Design review of the part built by this model. Coordinates are the model's own, in mm. A direction names the side the tool comes from. Coordinates: 2 decimals unless noted, no trailing zeros. Write each loop counter-clockwise with the first axis right and the second up, starting at its lowest first coordinate (ties: lowest second). Pieces come first, ordered by that corner, then holes. Notation, with made-up numbers: (85, 10) - (116, 10) arc R29 ccw to (116, 40) - close; hole circle Ø9 at (-28.75, 23). An arc over 180 degrees is marked (long way). One line per item, written item: value.
from build123d import *

# Parameters (mm, degrees)
SWEEP2_PROFILE_R     = 31.5
BOSS_EXTRUDE2_DEPTH  = 21
CUT_EXTRUDE4_REACH   = 47.019
SWEEP4_PROFILE_R     = 17.5
CUT_EXTRUDE5_START   = 2.5
CUT_EXTRUDE5_DEPTH   = 18.5
BOSS_EXTRUDE5_START  = 21
SKETCH47_R           = 5
BOSS_EXTRUDE5_DEPTH  = 7
BOSS_EXTRUDE6_START  = -21
SKETCH47_3_R         = 5
BOSS_EXTRUDE6_DEPTH  = 7
CUT_SWEEP1_PROFILE_R = 26
CUT_SWEEP2_PROFILE_R = 12


with BuildPart() as part:
    # Sweep2: sweep along a path in Sketch1
    with BuildLine(Plane.XY) as sweep2_path:
        Line((0, 35), (0, -35))
    # Sweep2 profile (on start of the path) → Sweep2 (sweep)
    with BuildSketch(Plane(origin=(0, 35, 0), x_dir=(-1, 0, 0), z_dir=(0, -1, 0))):
        Circle(SWEEP2_PROFILE_R)
    sweep(path=sweep2_path.line)

    # Sketch22 → Boss-Extrude2 (add, symmetric)
    with BuildSketch(Plane(origin=(0, 0, 0), x_dir=(1, 0, 0), z_dir=(0, 1, 0))):
        Polygon((0, 13), (240, 9), (240, -9), (0, -13), align=None)
    extrude(amount=BOSS_EXTRUDE2_DEPTH, both=True)

    # Sketch34 → Cut-Extrude4 (cut, up to next)
    with BuildSketch(Plane(origin=(0.216606498, 0, 12.996389892), x_dir=(0.99986114, 0, -0.016664352), z_dir=(0.016664352, 0, 0.99986114)), mode=Mode.PRIVATE) as cut_extrude4_sk1:
        with BuildLine():
            Line((87, 21), (243, 21))
            Line((243, 21), (243, 9))
            Line((243, 9), (128.569219382, 9))
            ThreePointArc((128.569219382, 9), (106.935911729, 12.060024019), (87, 21))
        make_face()
    cut_extrude4_tool1 = extrude(cut_extrude4_sk1.sketch, amount=-CUT_EXTRUDE4_REACH, mode=Mode.PRIVATE) & part.part
    add(cut_extrude4_tool1.solids().sort_by_distance((171.561444, 15.230505, 10.140643))[0], mode=Mode.SUBTRACT)
    # Sketch34 → Cut-Extrude4 (cut, up to next)
    with BuildSketch(Plane(origin=(0.216606498, 0, 12.996389892), x_dir=(0.99986114, 0, -0.016664352), z_dir=(0.016664352, 0, 0.99986114)), mode=Mode.PRIVATE) as cut_extrude4_sk2:
        with BuildLine():
            Line((128.569219382, -9), (243, -9))
            Line((243, -9), (243, -21))
            Line((243, -21), (87, -21))
            ThreePointArc((87, -21), (106.935911729, -12.060024019), (128.569219382, -9))
        make_face()
    cut_extrude4_tool2 = extrude(cut_extrude4_sk2.sketch, amount=-CUT_EXTRUDE4_REACH, mode=Mode.PRIVATE) & part.part
    add(cut_extrude4_tool2.solids().sort_by_distance((171.561444, -15.230505, 10.140643))[0], mode=Mode.SUBTRACT)

    # Sweep4: sweep along a path in Sketch35
    with BuildLine(Plane.XY) as sweep4_path:
        Line((250, 21), (250, -21))
    # Sweep4 profile (on start of the path) → Sweep4 (sweep)
    with BuildSketch(Plane(origin=(250, 21, 0), x_dir=(0, 0, -1), z_dir=(0, -1, 0))):
        Circle(SWEEP4_PROFILE_R)
    sweep(path=sweep4_path.line)

    # Sketch43 → Cut-Extrude5 (cut)
    with BuildSketch(Plane(origin=(0, 0, 0), x_dir=(1, 0, 0), z_dir=(0, 1, 0)).offset(CUT_EXTRUDE5_START)):
        with BuildLine():
            Line((70, 6), (220, 6))
            ThreePointArc((220, 6), (226, 0), (220, -6))
            Line((220, -6), (70, -6))
            ThreePointArc((70, -6), (64, 0), (70, 6))
        make_face()
    cut_extrude5 = extrude(amount=CUT_EXTRUDE5_DEPTH, mode=Mode.SUBTRACT)

    # Mirror2: Cut-Extrude5 across plane
    add(cut_extrude5.mirror(Plane.ZX), mode=Mode.SUBTRACT)

    # Sketch47 → Boss-Extrude5 (add)
    with BuildSketch(Plane(origin=(0, 0, 0), x_dir=(1, 0, 0), z_dir=(0, 1, 0)).offset(BOSS_EXTRUDE5_START)):
        with BuildLine():
            Line((87, -6), (87, -11.55))
            ThreePointArc((87, -11.55), (51.726774535, -22.345969003), (26.429629343, -49.193833472))
            ThreePointArc((26.429629343, -49.193833472), (17.766830002, -55.702151461), (7.181946677, -53.386435492))
            ThreePointArc((7.181946677, -53.386435492), (-14.855989459, -42.122318837), (-39.406288617, -38.986435492))
            ThreePointArc((-39.406288617, -38.986435492), (-50.326951915, -33.896458963), (-52.376901133, -22.023529412))
            ThreePointArc((-52.376901133, -22.023529412), (-48.925892025, 0), (-52.376901133, 22.023529412))
            ThreePointArc((-52.376901133, 22.023529412), (-50.326951915, 33.896458963), (-39.406288617, 38.986435492))
            ThreePointArc((-39.406288617, 38.986435492), (-14.855989459, 42.122318837), (7.181946677, 53.386435492))
            ThreePointArc((7.181946677, 53.386435492), (17.766830002, 55.702151461), (26.429629343, 49.193833472))
            ThreePointArc((26.429629343, 49.193833472), (51.726774535, 22.345969003), (87, 11.55))
            Line((87, 11.55), (86.912082494, 6))
            Line((86.912082494, 6), (70, 6))
            ThreePointArc((70, 6), (64, 0), (70, -6))
            Line((70, -6), (87, -6))
        make_face()
        with Locations((15, 43)):
            Circle(SKETCH47_R, mode=Mode.SUBTRACT)
        with Locations((-40, 26)):
            Circle(SKETCH47_R, mode=Mode.SUBTRACT)
        with Locations((-40, -26)):
            Circle(SKETCH47_R, mode=Mode.SUBTRACT)
        with Locations((15, -43)):
            Circle(SKETCH47_R, mode=Mode.SUBTRACT)
    extrude(amount=-BOSS_EXTRUDE5_DEPTH)

    # Sketch47<3> → Boss-Extrude6 (add)
    with BuildSketch(Plane(origin=(0, 0, 0), x_dir=(1, 0, 0), z_dir=(0, 1, 0)).offset(BOSS_EXTRUDE6_START)):
        with BuildLine():
            Line((87, -6), (87, -11.55))
            ThreePointArc((87, -11.55), (51.726774535, -22.345969003), (26.429629343, -49.193833472))
            ThreePointArc((26.429629343, -49.193833472), (17.766830002, -55.702151461), (7.181946677, -53.386435492))
            ThreePointArc((7.181946677, -53.386435492), (-14.855989459, -42.122318837), (-39.406288617, -38.986435492))
            ThreePointArc((-39.406288617, -38.986435492), (-50.326951915, -33.896458963), (-52.376901133, -22.023529412))
            ThreePointArc((-52.376901133, -22.023529412), (-48.925892025, 0), (-52.376901133, 22.023529412))
            ThreePointArc((-52.376901133, 22.023529412), (-50.326951915, 33.896458963), (-39.406288617, 38.986435492))
            ThreePointArc((-39.406288617, 38.986435492), (-14.855989459, 42.122318837), (7.181946677, 53.386435492))
            ThreePointArc((7.181946677, 53.386435492), (17.766830002, 55.702151461), (26.429629343, 49.193833472))
            ThreePointArc((26.429629343, 49.193833472), (51.726774535, 22.345969003), (87, 11.55))
            Line((87, 11.55), (86.912082494, 6))
            Line((86.912082494, 6), (70, 6))
            ThreePointArc((70, 6), (64, 0), (70, -6))
            Line((70, -6), (87, -6))
        make_face()
        with Locations((15, 43)):
            Circle(SKETCH47_3_R, mode=Mode.SUBTRACT)
        with Locations((-40, 26)):
            Circle(SKETCH47_3_R, mode=Mode.SUBTRACT)
        with Locations((-40, -26)):
            Circle(SKETCH47_3_R, mode=Mode.SUBTRACT)
        with Locations((15, -43)):
            Circle(SKETCH47_3_R, mode=Mode.SUBTRACT)
    extrude(amount=BOSS_EXTRUDE6_DEPTH)

    # Cut-Sweep1: sweep along a path in Sketch1<4>
    with BuildLine(Plane.XY) as cut_sweep1_path:
        Line((0, 35), (0, -35))
    # Cut-Sweep1 profile (on start of the path) → Cut-Sweep1 (sweep, cut)
    with BuildSketch(Plane(origin=(0, 35, 0), x_dir=(-1, 0, 0), z_dir=(0, -1, 0))):
        Circle(CUT_SWEEP1_PROFILE_R)
    sweep(path=cut_sweep1_path.line, mode=Mode.SUBTRACT)

    # Cut-Sweep2: sweep along a path in Sketch35<2>
    with BuildLine(Plane.XY) as cut_sweep2_path:
        Line((250, 21), (250, -21))
    # Cut-Sweep2 profile (on start of the path) → Cut-Sweep2 (sweep, cut)
    with BuildSketch(Plane(origin=(250, 21, 0), x_dir=(0, 0, -1), z_dir=(0, -1, 0))):
        Circle(CUT_SWEEP2_PROFILE_R)
    sweep(path=cut_sweep2_path.line, mode=Mode.SUBTRACT)


solid = part.part
1. For faces 1 (the face through (129, -8, 6)), 2 (the face through (52.171, -17.549, 22.072)), 3 (the face through (64, 12, 0)), list the 3-axis set-ups (+Z, -Z, +X, -X, +Y, -Y) from which the entire face can be reached by the end or side of a thin tool; tool diameter is ignored.
Answer block:
face 1: -Y
face 2: +Z, +Y, -Y
face 3: +Y
2. Consider section C-C, the plane x = 180.5. Write out the cut boundary in (y, z), then the cut area to 3 significant figures.
Answer block:
outline: (-9, -9.99) - (9, -9.99) - (9, -6) - (2.5, -6) - (2.5, 6) - (9, 6) - (9, 9.99) - (-9, 9.99) - (-9, 6) - (-2.5, 6) - (-2.5, -6) - (-9, -6) - close
area: 204 mm^2
3. Consider section A-A, the plane y = -5.5. Write out the cut boundary in (x, z).
Answer block:
outline: (28.91, -12.52) - (235.04, -9.08) arc R17.5 ccw (long way) to (235.04, 9.08) - (28.91, 12.52) arc R31.5 ccw (long way) to start; hole circle Ø52 at (0, 0); hole (70, -6) - (220, -6) arc R6 ccw to (220, 6) - (70, 6) arc R6 ccw to start; hole circle Ø24 at (250, 0)
4. Insertion check: pin 1 Ø6 at (y, z) = (23, -17.5) entering from +X; pin 2 Ø11.5 at (x, z) = (-40, 26) entering from +Y; pin 3 Ø17.5 at (x, z) = (249.5, 5) entering from -Y; pin 4 Ø9 at (x, z) = (-40, -26) entering from -Y. Each pin has a flat end and moves straight along its axis. Give the tip position at first contact, or say it passes through.
Answer block:
pin 1: stops at x = 258.56
pin 2: stops at y = 21
pin 3: stops at y = -21
pin 4: passes through
5. Mouldability with a two-part tool opening along Y and no side actions: class faces 4 (the face through (226, -6, 0)), 5 (the face through (26, -35, -5)), 6 (the face through (2, 14, 33)), 7 (the face through (107.1, 11.975, -8.721)) as released by +Y, released by -Y, zero draft, split by the parting line, or undercut.
Answer block:
face 4: zero draft
face 5: released by -Y
face 6: undercut
face 7: released by +Y
6. Wall thickness on line 1 along Z through (x, y) = (-40, -15.25); line 2 along Y through (x, z) = (-23.5, 36.5); line 3 along Z through (x, y) = (15, 19): over which ranges is each line inside the solid? List them lowest first.
Answer block:
line 1: z = -39 to -31, -21 to 21, 31 to 39
line 2: y = -21 to -14, 14 to 21
line 3: z = -56 to -48, -38 to -21.24, 21.24 to 38, 48 to 56
7. Consider section D-D, the plane y = -28. Write out the cut boundary in (x, z).
Answer block:
outline: circle Ø63 at (0, 0); hole circle Ø52 at (0, 0)
8. Consider section B-B, the plane z = 0. Give the number of separate pieces and of enclosed holes in the cut face, then the cut area to 3 significant figures.
Answer block:
separate pieces: 3
enclosed holes: 0
area: 3,770 mm^2
